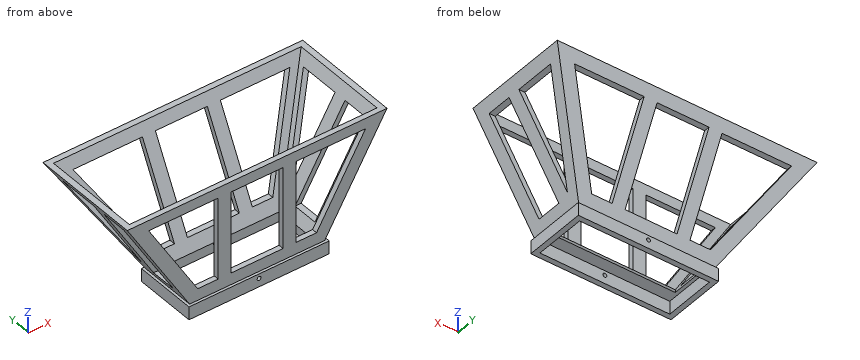
```python
from build123d import *

# Parameters (mm, degrees)
SKETCH_1_W          = 108
SKETCH_1_H          = 48
SKETCH_1_W_2        = 100
SKETCH_1_H_2        = 40
EXTRUDE_1_DEPTH     = 10
SKETCH_6_W          = 40
SKETCH_6_H          = 63
CUT_EXTRUDE_1_DEPTH = 102
SKETCH_7_W          = 64
SKETCH_7_H          = 20
CUT_EXTRUDE_2_DEPTH = 199
SKETCH_8_R          = 1.5
CUT_EXTRUDE_3_DEPTH = 139


with BuildPart() as part:
    # 草图1 → 凸台-拉伸1 (new body)
    with BuildSketch(Plane.XY):
        Rectangle(SKETCH_1_W, SKETCH_1_H)
        Rectangle(SKETCH_1_W_2, SKETCH_1_H_2, mode=Mode.SUBTRACT)
    extrude(amount=EXTRUDE_1_DEPTH)

    # 草图5 → 放样3 section 0
    with BuildSketch(Plane.XY.offset(90)):
        with BuildLine():
            Line((-100, -22), (100, -22))
            Line((100, -22), (100, 63))
            Line((100, 63), (-100, 63))
            Line((-100, 63), (-100, -22))
        make_face()
    # 草图2 → 放样3 section 1
    with BuildSketch(Plane.XY.offset(10)):
        with BuildLine():
            Line((52, 22), (-52, 22))
            Line((-52, 22), (-52, -22))
            Line((-52, -22), (52, -22))
            Line((52, -22), (52, 22))
        make_face()
    loft()

    # 抽壳2: read off the stored shape, not the designer's step
    # 抽壳2: loft between two sections, ruled curve by curve
    shell_2_from = [
        Edge.make_line((95.335238484, -18, 90), (95.335238484, 58.505280876, 90)),
        Edge.make_line((95.335238484, 58.505280876, 90), (-95.335238484, 58.505280876, 90)),
        Edge.make_line((-95.335238484, -18, 90), (95.335238484, -18, 90)),
        Edge.make_line((-95.335238484, 58.505280876, 90), (-95.335238484, -18, 90)),
    ]
    shell_2_to = [
        Edge.make_line((47.335238484, -18, 10), (47.335238484, 17.505280876, 10)),
        Edge.make_line((47.335238484, 17.505280876, 10), (-47.335238484, 17.505280876, 10)),
        Edge.make_line((-47.335238484, -18, 10), (47.335238484, -18, 10)),
        Edge.make_line((-47.335238484, 17.505280876, 10), (-47.335238484, -18, 10)),
    ]
    shell_2 = Solid(Shell([*[Face.make_surface_from_curves(shell_2_from[k], shell_2_to[k]) for k in range(4)], Face(Wire(shell_2_from)), Face(Wire(shell_2_to))]))
    add(shell_2, mode=Mode.SUBTRACT)

    # 草图6 → 切除-拉伸1 (cut)
    with BuildSketch(Plane.XZ.offset(24)):
        with Locations((0, 50.5)):
            Rectangle(SKETCH_6_W, SKETCH_6_H)
        Polygon((30, 19), (30, 82), (83.53809621, 82), (45.73809621, 19), align=None)
        Polygon((-45.73809621, 19), (-30, 19), (-30, 82), (-83.53809621, 82), align=None)
    extrude(amount=-CUT_EXTRUDE_1_DEPTH, mode=Mode.SUBTRACT)

    # 草图7 → 切除-拉伸2 (cut, symmetric)
    with BuildSketch(Plane.ZY.offset(54)):
        with Locations((50, -2)):
            Rectangle(SKETCH_7_W, SKETCH_7_H)
        Polygon((82, 49.910561753), (19.735489263, 18), (82, 18), align=None)
    extrude(amount=CUT_EXTRUDE_2_DEPTH, both=True, mode=Mode.SUBTRACT)

    # 草图8 → 切除-拉伸3 (cut)
    with BuildSketch(Plane(origin=(0, 24, 0), x_dir=(1, 0, 0), z_dir=(0, 1, 0))):
        with Locations(Location((0, -6.5, 0), (0, 0, 180))):
            Circle(SKETCH_8_R)
    extrude(amount=-CUT_EXTRUDE_3_DEPTH, mode=Mode.SUBTRACT)

    # 草图13 → 放样5 section 0
    with BuildSketch(Plane(origin=(30.393557709, 0, -18.236134625), x_dir=(0.5144957554275269, 0, 0.857492925712544), z_dir=(-0.857492925712544, 0, 0.5144957554275269))):
        with BuildLine():
            Line((32.928708539, -11), (43.42442195, -18))
            Line((43.42442195, -18), (32.928708539, -18))
            Line((32.928708539, -18), (32.928708539, -11))
        make_face()
    # 草图12 → 放样5 section 1
    with BuildSketch(Plane(origin=(-30.393557709, 0, -18.236134625), x_dir=(0.5144957554275263, 0, -0.8574929257125443), z_dir=(0.8574929257125443, 0, 0.5144957554275263))):
        with BuildLine():
            Line((-32.928708539, -11), (-43.42442195, -18))
            Line((-43.42442195, -18), (-32.928708539, -18))
            Line((-32.928708539, -18), (-32.928708539, -11))
        make_face()
    loft()


solid = part.part
```
Model file for the job. Use its own axes, mm. Round coordinates to 2 decimals unless told otherwise and drop trailing zeros. Put each result on its own line as item: value. Start each with the question number.
Item 1: Drill centre lines: line 1 along Z through (x, y) = (0, -21.4); line 2 along Z through (x, y) = (0, 22.7); line 3 along Z through (x, y) = (0, -23). Where is each one in solid material? Low to high.
Item 2: Cut at A-A (y = -2). Give the number of separate pieces and of enclosed holes in the cut face, then the cut area to 3 significant figures.
Item 3: Drop flat-ended pins along their axis: P1, Ø1.2, axis at x = 59.5, y = -19, coming from the -Z side; P2, Ø2, axis at y = 11.5, z = 47, coming from the +X side; P3, Ø8, axis at x = -23.5, z = 11.5, coming from the +Y side; P4, Ø2.5, axis at x = 0, z = 6.5, coming from the +Y side. Give the stop position or say it passes through.
Answer block:
1. line 1: 0 to 5, 8 to 19, 82 to 90
1. line 2: 0 to 5, 8 to 10, 11.37 to 19
1. line 3: 0 to 5, 8 to 10
2. separate pieces: 4
2. enclosed holes: 0
2. area: 229 mm2
3. P1: z = 21.5
3. P2: x = 74.8
3. P3: y = 24.82
3. P4: through
